Work out the finished part from the listing and answer in its coordinate system (mm). A direction names the side the tool comes from. Round coordinates to 2 decimals unless told otherwise and drop trailing zeros. Loops run counter-clockwise (first coordinate to the right, second up) from the corner with the lowest first, then second, coordinate; pieces in that order, holes last.
from build123d import *

# Parameters (mm, degrees)
SKETCH1_W           = 40
SKETCH1_H           = 40
SKETCH1_R           = 2.5
SKETCH1_R_2         = 16
BOSS_EXTRUDE1_DEPTH = 20
FILLET2_R           = 3
SKETCH7_W           = 18
SKETCH7_H           = 3
LPATTERN1_COUNT     = 5
LPATTERN1_PITCH     = 5.25
SKETCH8_R           = 10
CUT_EXTRUDE1_DEPTH  = 70
SKETCH10_W          = 12
SKETCH10_H          = 32
SKETCH10_R          = 3
BOSS_EXTRUDE2_DEPTH = 6
FILLET4_R           = 1.5


with BuildPart() as part:
    # Sketch1 → Boss-Extrude1 (new body, symmetric)
    with BuildSketch(Plane.XY):
        with Locations((0.017734769, -0.034630907)):
            Rectangle(SKETCH1_W, SKETCH1_H)
        with Locations((-14.982265231, 14.965369093)):
            Circle(SKETCH1_R, mode=Mode.SUBTRACT)
        with Locations((15.017734769, 14.965369093)):
            Circle(SKETCH1_R, mode=Mode.SUBTRACT)
        with Locations((15.017734769, -15.034630907)):
            Circle(SKETCH1_R, mode=Mode.SUBTRACT)
        with Locations((-14.982265231, -15.034630907)):
            Circle(SKETCH1_R, mode=Mode.SUBTRACT)
        with Locations((0.017734769, -0.034630907)):
            Circle(SKETCH1_R_2, mode=Mode.SUBTRACT)
    extrude(amount=BOSS_EXTRUDE1_DEPTH, both=True)

    # Fillet2
    fillet2_edges = [part.edges().sort_by_distance(p)[0] for p in [
        (20.017734769, -20.034630907, 0),
        (-19.982265231, -20.034630907, 0),
        (-19.982265231, 19.965369093, 0),
        (20.017734769, 19.965369093, 0),
    ]]
    fillet(fillet2_edges, radius=FILLET2_R)

    # Sketch2 → Revolve2 (revolve)
    with BuildSketch(Plane.XY):
        Polygon((0.017734769, 19.965369093), (0.017734769, 69.965369093), (-21.982265231, 69.965369093), (-17.982265231, 39.965369093), (-14.982265231, 39.965369093), (-14.982265231, 19.965369093), align=None)
    revolve(axis=Axis((0.017734769, 19.965369093, 0), (0, 1, 0)))

    # Sketch7 → Cut-Revolve3 (revolve, cut)
    with BuildSketch(Plane.XY):
        with Locations((-20.982265231, 44.465369093)):
            Rectangle(SKETCH7_W, SKETCH7_H)
    cut_revolve3 = revolve(axis=Axis((0.017734769, 42.965369093, 0), (0, 1, 0)), mode=Mode.SUBTRACT)

    # LPattern1: Cut-Revolve3 ×5
    with Locations(*[(0, i * LPATTERN1_PITCH, 0) for i in range(1, LPATTERN1_COUNT)]):
        add(cut_revolve3, mode=Mode.SUBTRACT)

    # Sketch8 → Cut-Extrude1 (cut)
    with BuildSketch(Plane(origin=(0, 69.965369093, 0), x_dir=(1, 0, 0), z_dir=(0, 1, 0))):
        with Locations((0.017734769, 0)):
            Circle(SKETCH8_R)
    extrude(amount=-CUT_EXTRUDE1_DEPTH, mode=Mode.SUBTRACT)

    # Sketch10 → Boss-Extrude2 (add)
    with BuildSketch(Plane(origin=(0, 0, 0), x_dir=(1, 0, 0), z_dir=(0, 1, 0))):
        with Locations((-25.982265231, 0.712845565)):
            Rectangle(SKETCH10_W, SKETCH10_H)
        with Locations((-26, -9)):
            Circle(SKETCH10_R, mode=Mode.SUBTRACT)
        with Locations((-26, 9)):
            Circle(SKETCH10_R, mode=Mode.SUBTRACT)
    boss_extrude2 = extrude(amount=BOSS_EXTRUDE2_DEPTH)

    # Mirror1: Boss-Extrude2 across plane
    add(boss_extrude2.mirror(Plane(origin=(0, 0, 0), x_dir=(0, 0, 1), z_dir=(1, 0, 0))))

    # Fillet4
    fillet4_edges = [part.edges().sort_by_distance(p)[0] for p in [
        (20.017734769, 0, -0.712845565),
        (20.017734769, 6, -0.712845565),
        (20.017734769, 3, 15.287154435),
        (26, 0, 15.287154435),
        (20.017734769, 3, -16.712845565),
        (31.982265231, 3, 15.287154435),
        (31.982265231, 3, -16.712845565),
        (26, 6, -16.712845565),
        (31.982265231, 6, -0.712845565),
        (26, 6, 15.287154435),
        (15.017734769, 19.965369093, 0),
        (-19.982265231, 6, -0.712845565),
        (-19.982265231, 3, -16.712845565),
        (-31.982265231, 3, -16.712845565),
        (-19.982265231, 3, 15.287154435),
        (-31.982265231, 3, 15.287154435),
        (-25.982265231, 6, -16.712845565),
        (-25.982265231, 6, 15.287154435),
        (-31.982265231, 6, -0.712845565),
    ]]
    fillet(fillet4_edges, radius=FILLET4_R)


solid = part.part
Item 1: Section B-B, the plane y = 3.5 is taken. Give the vertices of the cut face in (x, z), plus the area to 3 significant figures.
Item 2: Section D-D, the plane z = 11 is taken. State how many separate pieces and enclosed holes the cut face has, plus the area to 3 significant figures.
Item 3: For faces 1 (the face through (-26, 0, -1)), 2 (the face through (-9, 14, -20)), 3 (the face through (-31.982, 2, -1)), 4 (the face through (-26, 2, -16.713)), 5 (the face through (-9, 58.715, -9)), determine the directions among +Z, -Z, +X, -X, +Y, -Y from which every point of the face is accessible in a straight line to the end or side of a thin tool.
Item 4: Determine the mould class of faces 6 (the face through (-2.15, 41.613, 9.762)), 7 (the face through (9.54, 54.99, -7.3)), 8 (the face through (4, 39.965, 15)) for opening direction X: pulls with the +X half, pulls with the -X half, needs draft (parallel to the pull), parting line crosses it, or undercut.
Item 5: Section C-C, the plane x = -26 is taken. Give the vertices of the cut face in (y, z).
Item 6: Each of these flat-tipped pins is pushed along its axis until it touches: P1, Ø5.5, axis at x = 26, z = 9, coming from the +Y side; P2, Ø8.5, axis at x = 25, z = -2, coming from the -Y side; P3, Ø12, axis at x = 9.5, y = -8.5, coming from the +Z side; P4, Ø1, axis at x = -6, y = 46.5, coming from the -Z side. Where does it stop, or does it pass through?
Item 7: Section A-A, the plane x = 26 is taken. Give the vertices of the cut face in (y, z).
Item 8: Straight lines are drawn through the part: line 1 (Z direction, x = -26, y = 4); line 2 (X direction, y = 0.5, z = 13); line 3 (X direction, y = 17, z = 19.5). For each, find the intervals that lie inside material, in ascending order.
Answer below:
1. outline: (-31.98, -15.21) arc R1.5 ccw to (-30.48, -16.71) - (-21.48, -16.71) arc R1.5 cw to (-19.98, -18.21) - (-19.98, -20) - (-15.59, -20) - (-15.59, 20) - (-19.98, 20) - (-19.98, 16.79) arc R1.5 cw to (-21.48, 15.29) - (-30.48, 15.29) arc R1.5 ccw to (-31.98, 13.79) - close; (15.62, -20) - (20.02, -20) - (20.02, -18.21) arc R1.5 cw to (21.52, -16.71) - (30.48, -16.71) arc R1.5 ccw to (31.98, -15.21) - (31.98, 13.79) arc R1.5 ccw to (30.48, 15.29) - (21.52, 15.29) arc R1.5 cw to (20.02, 16.79) - (20.02, 20) - (15.62, 20) - close; hole circle Ø6 at (-26, -9); hole circle Ø6 at (-26, 9); hole circle Ø6 at (26, -9); hole circle Ø6 at (26, 9)
1. area: 1,010 mm2
2. separate pieces: 3
2. enclosed holes: 5
2. area: 1,850 mm2
3. face 1: +Z, -Z, -X, -Y
3. face 2: -Z, +X, -X, -Y
3. face 3: +Z, -Z, -X, +Y, -Y
3. face 4: -Z, -X, +Y, -Y
3. face 5: none
4. face 6: undercut
4. face 7: parting line crosses it
4. face 8: needs draft
5. outline: (0, -16.71) - (4.5, -16.71) arc R1.5 ccw to (6, -15.21) - (6, -12) - (0, -12) - close; (0, -6) - (6, -6) - (6, 6) - (0, 6) - close; (0, 12) - (6, 12) - (6, 13.79) arc R1.5 ccw to (4.5, 15.29) - (0, 15.29) - close
6. P1: passes through
6. P2: stops at y = -0.21
6. P3: stops at z = 20
6. P4: stops at z = -18.06
7. outline: (0, -16.71) - (4.5, -16.71) arc R1.5 ccw to (6, -15.21) - (6, -12) - (0, -12) - close; (0, -6) - (6, -6) - (6, 6) - (0, 6) - close; (0, 12) - (6, 12) - (6, 13.79) arc R1.5 ccw to (4.5, 15.29) - (1.5, 15.29) arc R1.5 ccw to (0, 13.79) - close
8. line 1: z = -16.71 to -12, -6 to 6, 12 to 15.29
8. line 2: x = -31.98 to -15.97, 16.01 to 31.98
8. line 3: x = -19.98 to -16.43, -13.53 to 13.57, 16.47 to 20.02
